The listing builds one solid part. Answer for the finished solid, in the listing's coordinates (mm). A direction names the side the tool comes from. Round coordinates to 2 decimals unless told otherwise and drop trailing zeros. Write each loop counter-clockwise with the first axis right and the second up, starting at its lowest first coordinate (ties: lowest second). Pieces come first, ordered by that corner, then holes. Notation, with made-up numbers: (64.5, -30.75) - (83.5, -30.75) arc R19 ccw to (83.5, -21.75) - close; hole circle Ø3 at (-22, 28). An arc over 180 degrees is marked (long way). Return JSON: item names as keys, results as strings. Group by question number.
(1) Find the intervals of material crossed by line 1 along Y through (x, z) = (26.5, 10.5); line 2 along X through (y, z) = (23.5, -5.5) (3 decimals), in increasing order. Write a range as [from, to].
(2) Which of the six approach directions +Z, -Z, +X, -X, +Y, -Y give full straight-line access (tool end or side, diameter ignored) to faces 1 (the flat face through (-25, 3, 6.74)), 2 (the flat face through (-16, 3.15, 14)), 3 (the cylindrical face through (-16.183, 2.39, 16.383)), 4 (the flat face through (7, 14, 20.105)), 5 (the flat face through (7, 14, -24.775))?
(3) Section D-D, the plane z = 6 is taken. Write down the section's boundary in (x, y) (3 decimals).
(4) Section B-B, the plane x = 10 is taken. Write down the section's boundary in (y, z) (3 decimals), then the cut area to 3 significant figures.
(5) Section C-C, the plane y = 12.75 is taken. Write down the section's boundary in (x, z) (3 decimals), then the cut area to 3 significant figures.
(6) Determine the mould class of faces 6 (the flat face through (-22.975, 3, 5)), 7 (the flat face through (34.515, 1, 0)), 8 (the flat face through (-27.415, 3, 13)), 9 (the flat face through (-25, 4.09, 13)) for opening direction X: +X half, -X half, draft (parallel to the pull), parting line (faces both ways), or undercut.
(7) Each of these flat-tipped pins is pushed along its axis until it touches: pin 1 (10 mm diameter, centred on y = 21.5, z = 17.5, fed in from -X) (3 decimals); pin 2 (2 mm diameter, centred on y = 2.5, z = 14, fed in from -X) (3 decimals); pin 3 (1.2 mm diameter, centred on x = -17, z = 7, fed in from +Y); pin 4 (2.5 mm diameter, centred on y = 3.5, z = 5.5, fed in from +X) (3 decimals). Where does it stop, or does it pass through?
(8) Section A-A, the plane z = -19 is taken. Write down the section's boundary in (x, y) (3 decimals), then the cut area to 3 significant figures.
```python
from build123d import *

# Parameters (mm, degrees)
SKETCH1_W             = 69.03
SKETCH1_H             = 54.27
BOSS_EXTRUDE1_DEPTH   = 1.65
SKETCH2_R             = 2
BOSS_EXTRUDE2_DEPTH   = 1.5
SKETCH3_W             = 4.44
SKETCH3_H             = 3.21
BOSS_EXTRUDE3_DEPTH   = 2.44
SKETCH4_W             = 17.82
SKETCH4_H             = 44.88
BOSS_EXTRUDE4_DEPTH   = 25
F_4_CLEARANCE_HOLE1_D = 2.8448


with BuildPart() as part:
    # Sketch1 → Boss-Extrude1 (new body)
    with BuildSketch(Plane(origin=(0, 0, 0), x_dir=(1, 0, 0), z_dir=(0, 1, 0))):
        Rectangle(SKETCH1_W, SKETCH1_H)
    extrude(amount=BOSS_EXTRUDE1_DEPTH)

    # Sketch2 → Boss-Extrude2 (add)
    with BuildSketch(Plane(origin=(0, 1.65, 0), x_dir=(1, 0, 0), z_dir=(0, 1, 0))):
        with Locations(Location((-16.095, -14.385, 0), (0, 0, 90))):
            Circle(SKETCH2_R)
        with Locations(Location((-16.095, -6.385, 0), (0, 0, 90))):
            Circle(SKETCH2_R)
    extrude(amount=BOSS_EXTRUDE2_DEPTH)

    # Sketch3 → Boss-Extrude3 (add)
    with BuildSketch(Plane(origin=(0, 1.65, 0), x_dir=(1, 0, 0), z_dir=(0, 1, 0))):
        with Locations((-25.195, -13.135)):
            Rectangle(SKETCH3_W, SKETCH3_H)
        with Locations((-25.195, -5.135)):
            Rectangle(SKETCH3_W, SKETCH3_H)
    extrude(amount=BOSS_EXTRUDE3_DEPTH)

    # Sketch4 → Boss-Extrude4 (add)
    with BuildSketch(Plane(origin=(0, 1.65, 0), x_dir=(1, 0, 0), z_dir=(0, 1, 0))):
        with Locations((6.925, 2.335)):
            Rectangle(SKETCH4_W, SKETCH4_H)
    extrude(amount=BOSS_EXTRUDE4_DEPTH)

    # #4 Clearance Hole1 (through all)
    with Locations(Plane(origin=(18.660321972, 1.65, 81.830440854), x_dir=(0, 0, 1), z_dir=(0, 1, 0))):
        with Locations((-106.465440854, -50.675321972), (-57.195440854, -50.675321972), (-57.195440854, 13.354678028), (-106.465440854, 13.354678028)):
            Hole(F_4_CLEARANCE_HOLE1_D / 2)


solid = part.part
```
Working result:
{
 "1": {"line 1": "y = [0, 1.65]", "line 2": "x = [-1.985, 15.835]"},
 "2": {"face 1": "-X, +Y", "face 2": "+Z, -Z, +Y", "face 3": "+Y", "face 4": "+Z, +X, -X, +Y", "face 5": "-Z, +X, -X, +Y"},
 "3": {"outline": "(-34.515, 0) - (34.515, 0) - (34.515, 1.65) - (15.835, 1.65) - (15.835, 26.65) - (-1.985, 26.65) - (-1.985, 1.65) - (-14.132, 1.65) - (-14.132, 3.15) - (-18.058, 3.15) - (-18.058, 1.65) - (-22.975, 1.65) - (-22.975, 4.09) - (-27.415, 4.09) - (-27.415, 1.65) - (-34.515, 1.65) - close"},
 "4": {"outline": "(0, -27.135) - (1.65, -27.135) - (1.65, -24.775) - (26.65, -24.775) - (26.65, 20.105) - (1.65, 20.105) - (1.65, 27.135) - (0, 27.135) - close", "area": "1,210 mm^2"},
 "5": {"outline": "(-1.985, -24.775) - (15.835, -24.775) - (15.835, 20.105) - (-1.985, 20.105) - close", "area": "800 mm^2"},
 "6": {"face 6": "undercut", "face 7": "+X half", "face 8": "-X half", "face 9": "draft"},
 "7": {"pin 1": "stops at x = -1.985", "pin 2": "stops at x = -34.515", "pin 3": "stops at y = 3.15", "pin 4": "stops at x = 15.835"},
 "8": {"outline": "(-34.515, 0) - (34.515, 0) - (34.515, 1.65) - (15.835, 1.65) - (15.835, 26.65) - (-1.985, 26.65) - (-1.985, 1.65) - (-34.515, 1.65) - close", "area": "559 mm^2"}
}
